```python
from build123d import *

# Parameters (mm, degrees)
BOSS_EXTRUDE1_DEPTH            = 15.24
SKETCH7_OUTSIDE_W              = 39.406
SKETCH7_OUTSIDE_H              = 20.102
CUT_EXTRUDE2_DEPTH             = 0.3048
F_2_56_TAPPED_HOLE1_AT_2_COUNT = 2
F_2_56_TAPPED_HOLE1_AT_2_PITCH = 24.13
F_31_0_12_DIAMETER_HOLE1_D     = 3.048
FILLET1_R                      = 1.016


with BuildPart() as part:
    # Sketch1 → Boss-Extrude1 (new, symmetric)
    with BuildSketch(Plane(origin=(0, 0, 0), x_dir=(0, 0, -1), z_dir=(1, 0, 0))):
        Polygon((5.588, 0), (-5.588, 0), (-5.588, -4.572), (2.032, -4.572), (2.032, -12.065), (5.588, -12.065), align=None)
    extrude(amount=BOSS_EXTRUDE1_DEPTH, both=True)

    # Sketch7 outside → Cut-Extrude2 (cut)
    with BuildSketch(Plane(origin=(0, 0, 0), x_dir=(1, 0, 0), z_dir=(0, 1, 0))):
        Rectangle(SKETCH7_OUTSIDE_W, SKETCH7_OUTSIDE_H)
        with BuildLine():
            Line((10.795, -4.191), (10.795, -5.08))
            ThreePointArc((10.795, -5.08), (10.646210245, -5.439210245), (10.287, -5.588))
            Line((10.287, -5.588), (-10.287, -5.588))
            ThreePointArc((-10.287, -5.588), (-10.646210245, -5.439210245), (-10.795, -5.08))
            Line((-10.795, -5.08), (-10.795, -4.191))
            ThreePointArc((-10.795, -4.191), (-10.646210245, -3.831789755), (-10.287, -3.683))
            Line((-10.287, -3.683), (10.287, -3.683))
            ThreePointArc((10.287, -3.683), (10.646210245, -3.831789755), (10.795, -4.191))
        make_face(mode=Mode.SUBTRACT)
        with BuildLine():
            Line((-10.287, 3.683), (10.287, 3.683))
            ThreePointArc((10.287, 3.683), (10.646210245, 3.831789755), (10.795, 4.191))
            Line((10.795, 4.191), (10.795, 5.08))
            ThreePointArc((10.795, 5.08), (10.646210245, 5.439210245), (10.287, 5.588))
            Line((10.287, 5.588), (-10.287, 5.588))
            ThreePointArc((-10.287, 5.588), (-10.646210245, 5.439210245), (-10.795, 5.08))
            Line((-10.795, 5.08), (-10.795, 4.191))
            ThreePointArc((-10.795, 4.191), (-10.646210245, 3.831789755), (-10.287, 3.683))
        make_face(mode=Mode.SUBTRACT)
    extrude(amount=-CUT_EXTRUDE2_DEPTH, mode=Mode.SUBTRACT)

    # Sketch2 → #2-56 Tapped Hole1 (revolve, cut)
    with BuildSketch(Plane(origin=(-12.065, -0.3048, 0), x_dir=(0, 0, 1), z_dir=(1, 0, 0))):
        Polygon((0, 0), (0, 4.2672), (1.397, 4.2672), (0.889, 3.7592), (0.889, 0.508), (1.397, 0), align=None)
    f_2_56_tapped_hole1 = revolve(axis=Axis((-12.065, 6.0452, 0), (0, -1, 0)), mode=Mode.SUBTRACT)

    # #2-56 Tapped Hole1 at 2: #2-56 Tapped Hole1 ×2
    with Locations(*[(i * F_2_56_TAPPED_HOLE1_AT_2_PITCH, 0, 0) for i in range(1, F_2_56_TAPPED_HOLE1_AT_2_COUNT)]):
        add(f_2_56_tapped_hole1, mode=Mode.SUBTRACT)

    # #31 (0.12) Diameter Hole1 (through all)
    with Locations(Plane(origin=(-4.633152105, -2.095479982, -2.032), x_dir=(1, 0, 0), z_dir=(0, 0, 1))):
        with Locations((-4.891847895, -6.438920018), (14.158152105, -6.438920018)):
            Hole(F_31_0_12_DIAMETER_HOLE1_D / 2)

    # Fillet1
    fillet1_edges = [part.edges().sort_by_distance(p)[0] for p in [
        (-15.24, -2.4384, 5.588),
        (15.24, -2.4384, 5.588),
        (15.24, -6.1849, -5.588),
        (-15.24, -6.1849, -5.588),
    ]]
    fillet(fillet1_edges, radius=FILLET1_R)


solid = part.part
```
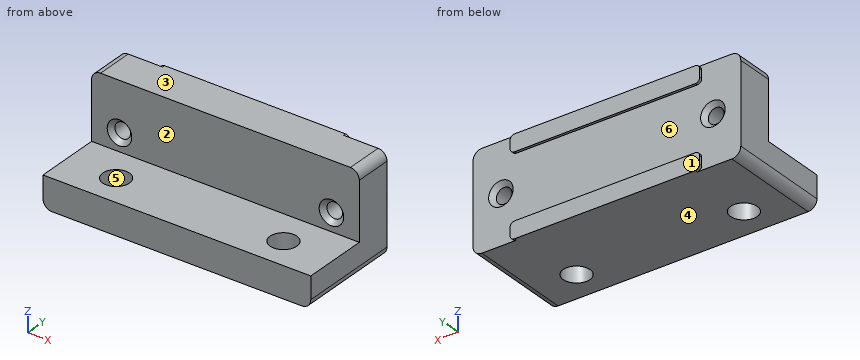
The model under review builds one solid part; all positions refer to its coordinate system, in mm. Face numbers are marked on the shaded views. A direction names the side the tool comes from. Round coordinates to 2 decimals unless told otherwise and drop trailing zeros. Order: outer loops, then holes, each group sorted by start corner. A loop starts at its lowest first (then second) coordinate and runs counter-clockwise, first axis right, second up. Notation, with made-up numbers: (-3, 13) - (52, 13) arc R17 ccw to (52, 39) - close; hole circle Ø4 at (-14, 22.5). An arc over 180 degrees is marked (long way). Answer in a Markdown table with one row per item.
(1) For line 1 (X direction, y = -1.7, z = 0); line 2 (Y direction, x = 0, z = 2.25); line 3 (Z direction, x = 3, y = -5.5), list the stretches that pass through material, from the lowest coordinate up. Write a range as from..to.
Result set:
| item | result |
|---|---|
| line 1 | x = -15.24..-12.95, -11.18..11.18, 12.95..15.24 |
| line 2 | y = -4.57..-0.3 |
| line 3 | z = -5.59..-2.03 |
(2) Clearance check with flat-ended pins moving along their axes: P1, Ø3.5, axis at x = -6.5, y = -7.5, coming from the +Z side; P2, Ø1.1, axis at x = 12.065, z = 0, coming from the +Y side; P3, Ø4, axis at x = -5, z = 0.5, coming from the -Y side; P4, Ø5.5, axis at x = 6, z = 2.5, coming from the +Y side. State where each tip first meets the part, or that it passes through.
Result set:
| item | result |
|---|---|
| P1 | stops at z = -2.03 |
| P2 | passes through |
| P3 | stops at y = -4.57 |
| P4 | stops at y = 0 |
(3) Machinability: for the marked faces 1 and 2, which of the approach directions +Z, -Z, +X, -X, +Y, -Y give a long, thin tool a straight path to every point of the face, cutting with its end or side? Answer none if there is none.
Result set:
| item | result |
|---|---|
| face 1 | +Z, -Z, +X, -X, +Y |
| face 2 | +Z, +X, -X, -Y |
(4) Take a section at C-C on x = 9. Write out the cut boundary in (y, z) (3 decimals).
Result set:
| item | result |
|---|---|
| outline | (-12.065, -5.588) - (-9.965, -5.588) - (-9.965, -2.032) - (-12.065, -2.032) - close; (-7.104, -5.588) - (0, -5.588) - (0, -3.683) - (-0.305, -3.683) - (-0.305, 3.683) - (0, 3.683) - (0, 5.588) - (-4.572, 5.588) - (-4.572, -2.032) - (-7.104, -2.032) - close |
(5) Take a section at A-A on z = 0. Write out the cut boundary in (x, y), plus the area to 3 significant figures.
Result set:
| item | result |
|---|---|
| outline | (-15.24, -4.57) - (-13.46, -4.57) - (-12.95, -4.06) - (-12.95, -0.81) - (-13.46, -0.3) - (-15.24, -0.3) - close; (-11.18, -4.06) - (-10.67, -4.57) - (10.67, -4.57) - (11.18, -4.06) - (11.18, -0.81) - (10.67, -0.3) - (-10.67, -0.3) - (-11.18, -0.81) - close; (12.95, -4.06) - (13.46, -4.57) - (15.24, -4.57) - (15.24, -0.3) - (13.46, -0.3) - (12.95, -0.81) - close |
| area | 114 mm2 |
(6) Take a section at B-B on y = -8.25. Write out the cut boundary in (x, z), plus the area to 3 significant figures.
Result set:
| item | result |
|---|---|
| outline | (-15.24, -4.57) arc R1.02 ccw to (-14.22, -5.59) - (-11.02, -5.59) - (-11.02, -2.03) - (-15.24, -2.03) - close; (-8.03, -5.59) - (8.03, -5.59) - (8.03, -2.03) - (-8.03, -2.03) - close; (11.02, -5.59) - (14.22, -5.59) arc R1.02 ccw to (15.24, -4.57) - (15.24, -2.03) - (11.02, -2.03) - close |
| area | 86.6 mm2 |
(7) Mouldability with a two-part tool opening along Z and no side actions: class the marked faces 3, 4, 5 and 6 as released by +Z, released by -Z, zero draft, split by the parting line, or undercut.
Result set:
| item | result |
|---|---|
| face 3 | released by +Z |
| face 4 | released by -Z |
| face 5 | zero draft |
| face 6 | undercut |
(8) Take a section at D-D on x = 1. Write out the cut boundary in (y, z) (3 decimals), plus the area to 3 significant figures.
Result set:
| item | result |
|---|---|
| outline | (-12.065, -5.588) - (0, -5.588) - (0, -3.683) - (-0.305, -3.683) - (-0.305, 3.683) - (0, 3.683) - (0, 5.588) - (-4.572, 5.588) - (-4.572, -2.032) - (-12.065, -2.032) - close |
| area | 75.5 mm2 |
